```python
from build123d import *

# Parameters (mm, degrees)
SKETCH_1_R      = 1.45
EXTRUDE_1_DEPTH = 3
FILLET_2_R      = 3


with BuildPart() as part:
    # 草图1 → 凸台-拉伸1 (new body)
    with BuildSketch(Plane(origin=(0, 0, 0), x_dir=(1, 0, 0), z_dir=(0, 1, 0))):
        Polygon((7.5, 31.5), (26.5, 7.5), (26.5, -7.5), (-26.5, -7.5), (-26.5, 7.5), (-7.5, 31.5), align=None)
        with Locations(Location((0, 26.5, 0), (0, 0, 270))):
            Circle(SKETCH_1_R, mode=Mode.SUBTRACT)
        with Locations(Location((0, 16.5, 0), (0, 0, 270))):
            Circle(SKETCH_1_R, mode=Mode.SUBTRACT)
        with Locations(Location((16.5, 0, 0), (0, 0, 270))):
            Circle(SKETCH_1_R, mode=Mode.SUBTRACT)
        with Locations(Location((-16.5, 0, 0), (0, 0, 270))):
            Circle(SKETCH_1_R, mode=Mode.SUBTRACT)
        Polygon((-7.5, 7.5), (-7.5, 26.666770148), (-22.673693034, 7.5), align=None, mode=Mode.SUBTRACT)
        Polygon((22.673693034, 7.5), (7.5, 7.5), (7.5, 26.666770148), align=None, mode=Mode.SUBTRACT)
    extrude(amount=EXTRUDE_1_DEPTH)

    # 圆角2
    fillet_2_edges = [part.edges().sort_by_distance(p)[0] for p in [
        (22.673693034, 1.5, -7.5),
        (7.5, 1.5, -26.666770148),
        (7.5, 1.5, -7.5),
        (26.5, 1.5, -7.5),
        (26.5, 1.5, 7.5),
        (-26.5, 1.5, 7.5),
        (-26.5, 1.5, -7.5),
        (-7.5, 1.5, -31.5),
        (7.5, 1.5, -31.5),
        (-7.5, 1.5, -26.666770148),
        (-22.673693034, 1.5, -7.5),
        (-7.5, 1.5, -7.5),
    ]]
    fillet(fillet_2_edges, radius=FILLET_2_R)


solid = part.part
```
Source: CAD feature listing. Evaluate the final solid. Frame: model axes, mm. A direction names the side the tool comes from. Give positions to 0.01 mm unless a question says otherwise; leave off trailing zeros. Loops run counter-clockwise (first coordinate to the right, second up) from the corner with the lowest first, then second, coordinate; pieces in that order, holes last. Notation, with made-up numbers: (34, -15) -> (40, -15) arc R20 ccw to (40, 11) -> close; hole circle Ø7 at (57, -10.5). An arc over 180 degrees is marked (long way). Use a Markdown table: item, result. Add a question column.
(1) Pull-direction query (X, two-part tool) for faces 1 (the face through (-14, 1, -7.5)), 2 (the face through (0, 0, -8)), 3 (the face through (26.329, 1.521, -7.455)); classes: +X half, -X half, draft (parallel to the pull), parting line (faces both ways), or undercut.
(2) Section query D-D (z = -26.5). Output: boundary loops of the cut face in (x, y).
(3) First-contact query: pin 1 Ø1.5 at (x, y) = (-14, 2) entering from -Z; pin 2 Ø0.9 at (y, z) = (1.5, -13.5) entering from +X. Flat tips, straight axial feed; report the tip coordinate or a pass-through.
(4) Ray query, line 1 (X direction, y = 1.5, z = 0); line 2 (X direction, y = 2.1, z = -18); line 3 (X direction, y = 2.5, z = -17). Return the intervals inside material, ascending.
(5) Access query for faces 4 (the face through (7.372, 1.521, -31.192)), 5 (the face through (14, 1, -7.5)). Directions: +Z, -Z, +X, -X, +Y, -Y. A direction counts if a zero-diameter tool reaches every point of the face in a straight line with its end or side. Return the directions, or none.
(6) Section query A-A (y = 0.9). Output: boundary loops of the cut face in (x, z), then the cut area to 3 significant figures.
(7) Section query C-C (z = -16.5). Output: boundary loops of the cut face in (x, y) (3 decimals), then the cut area to 3 significant figures.
(8) Section query B-B (z = 0). Output: boundary loops of the cut face in (x, y), then the cut area to 3 significant figures.
Checked values:
| question | item | result |
|---|---|---|
| 1 | face 1 | undercut |
| 1 | face 2 | draft |
| 1 | face 3 | +X half |
| 2 | outline | (-11.46, 0) -> (-1.45, 0) -> (-1.45, 3) -> (-11.46, 3) -> close; (1.45, 0) -> (11.46, 0) -> (11.46, 3) -> (1.45, 3) -> close |
| 3 | pin 1 | z = -24.24 |
| 3 | pin 2 | x = 22.11 |
| 4 | line 1 | -26.5 to -17.95, -15.05 to 15.05, 17.95 to 26.5 |
| 4 | line 2 | -18.19 to -14.36, -7.5 to 7.5, 14.36 to 18.19 |
| 4 | line 3 | -18.98 to -15.15, -7.5 to -1.36, 1.36 to 7.5, 15.15 to 18.98 |
| 5 | face 4 | -Z, +X, +Y, -Y |
| 5 | face 5 | +Y, -Y |
| 6 | outline | (-26.5, -6.46) arc R3 ccw to (-25.85, -8.32) -> (-8.4, -30.36) arc R3 ccw to (-6.05, -31.5) -> (6.05, -31.5) arc R3 ccw to (8.4, -30.36) -> (25.85, -8.32) arc R3 ccw to (26.5, -6.46) -> (26.5, 4.5) arc R3 ccw to (23.5, 7.5) -> (-23.5, 7.5) arc R3 ccw to (-26.5, 4.5) -> close; hole (-18.82, -12.36) -> (-12.85, -19.91) arc R3 ccw to (-7.5, -18.04) -> (-7.5, -10.5) arc R3 ccw to (-10.5, -7.5) -> (-16.47, -7.5) arc R3 ccw to start; hole circle Ø2.9 at (-16.5, 0); hole circle Ø2.9 at (0, -26.5); hole circle Ø2.9 at (0, -16.5); hole (7.5, -18.04) arc R3 ccw to (12.85, -19.91) -> (18.82, -12.36) arc R3 ccw to (16.47, -7.5) -> (10.5, -7.5) arc R3 ccw to (7.5, -10.5) -> close; hole circle Ø2.9 at (16.5, 0) |
| 6 | area | 1,340 mm^2 |
| 7 | outline | (-19.375, 0) -> (-15.549, 0) -> (-15.549, 3) -> (-19.375, 3) -> close; (-7.5, 0) -> (-1.45, 0) -> (-1.45, 3) -> (-7.5, 3) -> close; (1.45, 0) -> (7.5, 0) -> (7.5, 3) -> (1.45, 3) -> close; (15.549, 0) -> (19.375, 0) -> (19.375, 3) -> (15.549, 3) -> close |
| 7 | area | 59.3 mm^2 |
| 8 | outline | (-26.5, 0) -> (-17.95, 0) -> (-17.95, 3) -> (-26.5, 3) -> close; (-15.05, 0) -> (15.05, 0) -> (15.05, 3) -> (-15.05, 3) -> close; (17.95, 0) -> (26.5, 0) -> (26.5, 3) -> (17.95, 3) -> close |
| 8 | area | 142 mm^2 |
